Build history of the part. All positions in model axes, mm. Face numbers are marked on the shaded views. A direction names the side the tool comes from. Coordinates: 2 decimals unless noted, no trailing zeros. Order: outer loops, then holes, each group sorted by start corner. A loop starts at its lowest first (then second) coordinate and runs counter-clockwise, first axis right, second up. Notation, with made-up numbers: (28.5, 81.5) - (83.5, 81.5) arc R20 cw to (83.5, 116.5) - close; hole circle Ø11 at (32, 33.25). An arc over 180 degrees is marked (long way). One line per item, written item: value.
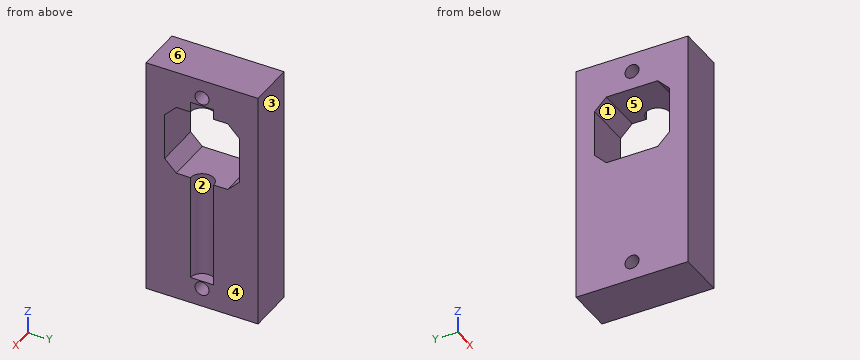
from build123d import *

# Parameters (mm, degrees)
SKETCH_1_W          = 42
SKETCH_1_H          = 42
EXTRUDE_1_DEPTH     = 40
CHAMFER_1_SIZE      = 5
SKETCH_4_R          = 1.75
CUT_EXTRUDE_1_DEPTH = 3
SKETCH_5_W          = 26
SKETCH_5_H          = 24
SKETCH_5_W_2        = 15
SKETCH_5_H_2        = 16
EXTRUDE_2_DEPTH     = 21
SKETCH_7_W          = 40
SKETCH_7_H          = 24
CUT_EXTRUDE_3_DEPTH = 21
SKETCH_6_R          = 3
CUT_EXTRUDE_2_DEPTH = 10
CHAMFER_2_SIZE      = 2.5
SKETCH_8_W          = 51.5
SKETCH_8_H          = 24
SKETCH_8_R          = 1.5
EXTRUDE_3_DEPTH     = 10
CUT_EXTRUDE_5_DEPTH = 73.374028491
CUT_EXTRUDE_START   = -5.8
SKETCH_10_R         = 2.5
CUT_EXTRUDE_6_DEPTH = 40


with BuildPart() as part:
    # Sketch 1 → Extrude 1 (new body)
    with BuildSketch(Plane.XY):
        Rectangle(SKETCH_1_W, SKETCH_1_H)
    extrude(amount=EXTRUDE_1_DEPTH)

    # Chamfer 1
    chamfer_1_edges = [part.edges().sort_by_distance(p)[0] for p in [
        (-21, 21, 20),
        (21, 21, 20),
        (21, -21, 20),
        (-21, -21, 20),
    ]]
    chamfer(chamfer_1_edges, length=CHAMFER_1_SIZE)

    # Sketch 4 → Cut-Extrude 1 (cut)
    with BuildSketch(Plane.XY.offset(40)):
        with Locations((-15.5, 15.5)):
            Circle(SKETCH_4_R)
        with Locations(Location((-15.5, -15.5, 0), (0, 0, 180))):
            Circle(SKETCH_4_R)
        with Locations((15.5, -15.5)):
            Circle(SKETCH_4_R)
        with Locations(Location((15.5, 15.5, 0), (0, 0, 180))):
            Circle(SKETCH_4_R)
    extrude(amount=-CUT_EXTRUDE_1_DEPTH, mode=Mode.SUBTRACT)

    # Sketch 7 → Cut-Extrude 3 (cut)
    with BuildSketch(Plane(origin=(21, 0, 0), x_dir=(0, 0, -1), z_dir=(1, 0, 0))):
        with Locations((-20, 0)):
            Rectangle(SKETCH_7_W, SKETCH_7_H)
    extrude(amount=-CUT_EXTRUDE_3_DEPTH, mode=Mode.SUBTRACT)


with BuildPart() as body_2:
    # Sketch 5 → Extrude 2 (new body)
    with BuildSketch(Plane.ZY.offset(21)):
        with Locations((53, 0)):
            Rectangle(SKETCH_5_W, SKETCH_5_H)
        with Locations((50.5, 0)):
            Rectangle(SKETCH_5_W_2, SKETCH_5_H_2, mode=Mode.SUBTRACT)
    extrude(amount=-EXTRUDE_2_DEPTH)


with BuildPart() as cut_extrude_2_tool:
    # Sketch 6 → Cut-Extrude 2 (new body)
    with BuildSketch(Plane(origin=(0, 0, 0), x_dir=(0, 0, -1), z_dir=(1, 0, 0))):
        with Locations((-62, 0)):
            Circle(SKETCH_6_R)
        with Locations((-18.5, 0)):
            Circle(SKETCH_6_R)
    extrude(amount=-CUT_EXTRUDE_2_DEPTH)


with BuildPart() as part_1:
    add(part.part)

    # Cut-Extrude 2: cut by cut_extrude_2_tool
    add(cut_extrude_2_tool.part, mode=Mode.SUBTRACT)



with BuildPart() as body_2_1:
    add(body_2.part)

    # Cut-Extrude 2: cut by cut_extrude_2_tool
    add(cut_extrude_2_tool.part, mode=Mode.SUBTRACT)

    # Chamfer 2
    chamfer_2_edges = [body_2_1.edges().sort_by_distance(p)[0] for p in [
        (-10.5, -8, 43),
        (-10.5, 8, 43),
        (-10.5, 8, 58),
        (-10.5, -8, 58),
    ]]
    chamfer(chamfer_2_edges, length=CHAMFER_2_SIZE)


with BuildPart() as part_2:
    add(part_1.part)

    add(body_2_1.part)  # Extrude 3 merges body 2
    # Sketch 8 → Extrude 3 (add)
    with BuildSketch(Plane(origin=(0, 0, 0), x_dir=(0, 0, -1), z_dir=(1, 0, 0))):
        with Locations((-40.25, 0)):
            Rectangle(SKETCH_8_W, SKETCH_8_H)
        with Locations((-62, 0)):
            Circle(SKETCH_8_R, mode=Mode.SUBTRACT)
        with Locations((-18.5, 0)):
            Circle(SKETCH_8_R, mode=Mode.SUBTRACT)
        Polygon((-58, 5.5), (-58, -5.5), (-55.5, -8), (-45.5, -8), (-43, -5.5), (-43, 5.5), (-45.5, 8), (-55.5, 8), align=None, mode=Mode.SUBTRACT)
    extrude(amount=EXTRUDE_3_DEPTH)

    # Sketch 9 → Cut-Extrude 5 (cut, through all)
    with BuildSketch(Plane.XY.offset(66)):
        Polygon((21, 12), (21, 16), (16, 21), (-16, 21), (-21, 16), (-21, -16), (-16, -21), (16, -21), (21, -16), (21, -12), (0, -12), (0, 12), align=None)
    extrude(amount=-CUT_EXTRUDE_5_DEPTH, mode=Mode.SUBTRACT)

    # Sketch 10 → Cut-Extrude 6 (cut)
    with BuildSketch(Plane.XY.offset(66).offset(CUT_EXTRUDE_START)):
        with Locations((10, 0)):
            Circle(SKETCH_10_R)
    extrude(amount=-CUT_EXTRUDE_6_DEPTH, mode=Mode.SUBTRACT)


solid = part_2.part
1. Band-saw the part on D-D, the plane y = 0. Give the cut face in (x, z), and give its area (4 significant figures).
Values found:
outline: (0, 14.5) - (10, 14.5) - (10, 17) - (0, 17) - close; (0, 20) - (10, 20) - (10, 20.2) - (7.5, 20.2) - (7.5, 43) - (0, 43) - close; (0, 58) - (7.5, 58) - (7.5, 60.2) - (10, 60.2) - (10, 60.5) - (0, 60.5) - close; (0, 63.5) - (10, 63.5) - (10, 66) - (0, 66) - close
area: 242.5 mm2
2. Flat gauge pin, fed straight in: P1, Ø6, axis at y = 5, z = 23.5, coming from the -X side. Where does the tip first touch, or does it go through?
Values found:
P1: stops at x = 0
3. Band-saw the part on C-C, the plane x = 4.75. Give the cut face in (y, z), and give its area (3 significant figures).
Values found:
outline: (-12, 14.5) - (12, 14.5) - (12, 66) - (-12, 66) - close; hole (-8, 45.5) - (-5.5, 43) - (5.5, 43) - (8, 45.5) - (8, 55.5) - (5.5, 58) - (-5.5, 58) - (-8, 55.5) - close; hole circle Ø3 at (0, 18.5); hole circle Ø3 at (0, 62)
area: 994 mm2
4. Probe line 1 along Z through (x, y) = (5, -4); line 2 along Y through (x, z) = (4, 49.5); line 3 along Y through (x, z) = (3, 62). List the from-to ranges inside material, lowest first.
Values found:
line 1: z = 14.5 to 43, 58 to 66
line 2: y = -12 to -8, 8 to 12
line 3: y = -12 to -1.5, 1.5 to 12
5. Band-saw the part on A-A, the plane y = 3.5. Give the cut face in (x, z), and give its area (3 significant figures).
Values found:
outline: (0, 14.5) - (10, 14.5) - (10, 43) - (0, 43) - close; (0, 58) - (10, 58) - (10, 66) - (0, 66) - close
area: 365 mm2
6. Two-plate mould, pull along Y, no slides. Class the marked faces 1, 2, 3 and 4: pulls with the +Y half, pulls with the -Y half, needs draft (parallel to the pull), parting line crosses it, or undercut.
Values found:
face 1: undercut
face 2: undercut
face 3: pulls with the +Y half
face 4: needs draft
7. Band-saw the part on B-B, the plane z = 18.5. Give the cut face in (x, y), and give its area (3 significant figures).
Values found:
outline: (0, -12) - (10, -12) - (10, -1.5) - (0, -1.5) - close; (0, 1.5) - (10, 1.5) - (10, 12) - (0, 12) - close
area: 210 mm2
8. 3-axis set-ups, long thin cutter, end or side, ignore diameter. For the marked faces 5 and 6: which of +Z, -Z, +X, -X, +Y, -Y reach the whole face in a straight line?
Values found:
face 5: +X, -X
face 6: +Z, +X, -X, +Y, -Y
